Job drawing, mm, ordinate dimensions from the low corner. One solid piece. A direction names the side the tool comes from. Round coordinates to 2 decimals unless told otherwise and drop trailing zeros. Loops run counter-clockwise (first coordinate to the right, second up) from the corner with the lowest first, then second, coordinate; pieces in that order, holes last.
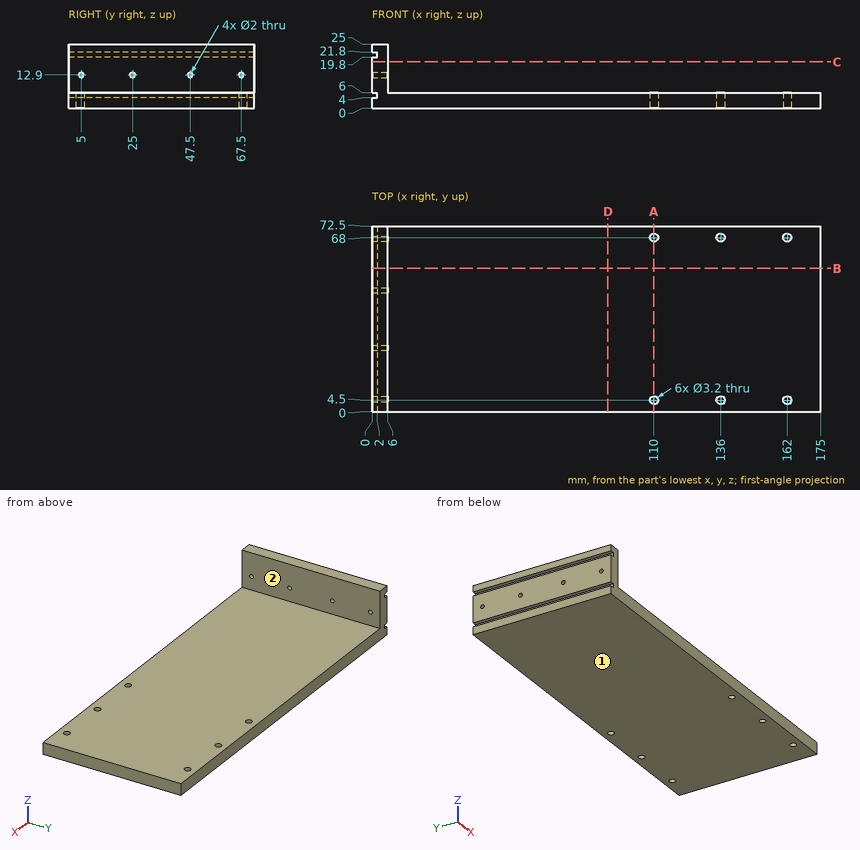
(1) Slice it at A-A on x = 110. List the corners of the cut face in (y, z), plus the area to 3 significant figures.
Responses:
outline: (0, 0) - (2.9, 0) - (2.9, 6) - (0, 6) - close; (6.1, 0) - (66.4, 0) - (66.4, 6) - (6.1, 6) - close; (69.6, 0) - (72.5, 0) - (72.5, 6) - (69.6, 6) - close
area: 397 mm2
(2) Which spindle directions (+Z, -Z, +X, -X, +Y, -Y) get a long thin tool onto all of the face, cutting with end or side? Do the marked faces 1 and 2. Say none if no direction does.
Responses:
face 1: -Z, +X, -X, +Y, -Y
face 2: +Z, +X, +Y, -Y
(3) Probe line 1 (Y direction, x = 162, z = 1.95); line 2 (X direction, y = 68, z = 3.8); line 3 (Z direction, x = 2.5, y = 67.5). List the from-to ranges inside material, lowest first.
Responses:
line 1: y = 0 to 2.9, 6.1 to 66.4, 69.6 to 72.5
line 2: x = 0 to 108.4, 111.6 to 134.4, 137.6 to 160.4, 163.6 to 175
line 3: z = 0 to 11.9, 13.9 to 25
(4) Slice it at D-D on x = 92. List the corners of the cut face in (y, z), plus the area to 3 significant figures.
Responses:
outline: (0, 0) - (72.5, 0) - (72.5, 6) - (0, 6) - close
area: 435 mm2
(5) Slice it at C-C on z = 18. List the corners of the cut face in (x, y), plus the area to 3 significant figures.
Responses:
outline: (0, 0) - (6, 0) - (6, 72.5) - (0, 72.5) - close
area: 435 mm2
(6) Slice it at B-B on y = 56. List the corners of the cut face in (x, z), plus the area to 3 significant figures.
Responses:
outline: (0, 0) - (175, 0) - (175, 6) - (6, 6) - (6, 25) - (0, 25) - (0, 21.8) - (2, 21.8) - (2, 19.8) - (0, 19.8) - (0, 6) - (2, 6) - (2, 4) - (0, 4) - close
area: 1,160 mm2
(7) Pin check, flat tips, straight feed: P1, Ø1.5, axis at x = 101.5, y = 46.5, coming from the +Z side; P2, Ø1.5, axis at y = 59, z = 21, coming from the -X side; P3, Ø5.5, axis at y = 53.5, z = 17, coming from the +X side. Stop position of each tip, or through.
Responses:
P1: stops at z = 6
P2: stops at x = 2
P3: stops at x = 6
